from build123d import *

# Parameters (mm, degrees)
BOSS_EXTRU_1_DEPTH      = 12
ESQUISSE2_R             = 2
ENL_V_MAT_EXTRU_1_DEPTH = 28.690963204
ESQUISSE4_R             = 3.7
ENL_V_MAT_EXTRU_2_DEPTH = 17


with BuildPart() as part:
    # Esquisse1 → Boss.-Extru.1 (new, symmetric)
    with BuildSketch(Plane.XY):
        with BuildLine():
            Line((15.300968977, -0.378320662), (15.300968977, 10.466871635))
            Line((15.300968977, 10.466871635), (0, 10.466871635))
            Line((0, 10.466871635), (0, 7.5))
            ThreePointArc((0, 7.5), (5.303300859, 5.303300859), (7.5, 0))
            ThreePointArc((7.5, 0), (5.303300859, -5.303300859), (0, -7.5))
            Line((0, -7.5), (0, -9.247838393))
            Line((0, -9.247838393), (5.044275487, -9.247838393))
            Line((5.044275487, -9.247838393), (15.300968977, -0.378320662))
        make_face()
        with BuildLine():
            Line((0, 7.5), (0, 10.466871635))
            Line((0, 10.466871635), (-15.300968977, 10.466871635))
            Line((-15.300968977, 10.466871635), (-15.300968977, -0.378320662))
            Line((-15.300968977, -0.378320662), (-5.044275487, -9.247838393))
            Line((-5.044275487, -9.247838393), (0, -9.247838393))
            Line((0, -9.247838393), (0, -7.5))
            ThreePointArc((0, -7.5), (-7.5, 0), (0, 7.5))
        make_face()
    extrude(amount=BOSS_EXTRU_1_DEPTH, both=True)

    # Esquisse2 → Enlèv. mat.-Extru.1 (cut, through all)
    with BuildSketch(Plane(origin=(0, 10.466871635, 0), x_dir=(1, 0, 0), z_dir=(0, 1, 0))):
        with Locations(Location((-11.300968977, 8, 0), (0, 0, 270))):
            Circle(ESQUISSE2_R)
        with Locations(Location((-11.300968977, -8, 0), (0, 0, 270))):
            Circle(ESQUISSE2_R)
        with Locations(Location((11.300968977, -8, 0), (0, 0, 270))):
            Circle(ESQUISSE2_R)
        with Locations(Location((11.300968977, 8, 0), (0, 0, 270))):
            Circle(ESQUISSE2_R)
    extrude(amount=-ENL_V_MAT_EXTRU_1_DEPTH, mode=Mode.SUBTRACT)

    # Esquisse4 → Enlèv. mat.-Extru.2 (cut)
    with BuildSketch(Plane.XZ.offset(9.247838393)):
        with Locations(Location((-11.300968977, 8, 0), (0, 0, 270))):
            Circle(ESQUISSE4_R)
        with Locations(Location((-11.300968977, -8, 0), (0, 0, 270))):
            Circle(ESQUISSE4_R)
        with Locations(Location((11.300968977, 8, 0), (0, 0, 270))):
            Circle(ESQUISSE4_R)
        with Locations(Location((11.300968977, -8, 0), (0, 0, 270))):
            Circle(ESQUISSE4_R)
    extrude(amount=-ENL_V_MAT_EXTRU_2_DEPTH, mode=Mode.SUBTRACT)


solid = part.part
Design review of the part built by this model. Coordinates are the model's own, in mm. A direction names the side the tool comes from. Coordinates: 2 decimals unless noted, no trailing zeros. Order: outer loops, then holes, each group sorted by start corner. A loop starts at its lowest first (then second) coordinate and runs counter-clockwise, first axis right, second up. Notation, with made-up numbers: (17.5, -1) -> (27.5, -1) arc R25 cw to (27.5, 38) -> close; hole circle Ø8 at (-27.75, -23.5). An arc over 180 degrees is marked (long way). One line per item, written item: value.
1) To check wall thickness, follow probe 1 along X at (y, z) = (9.95, -8); probe 2 along Z at (x, y) = (10, 5.5); probe 3 along Z at (x, y) = (-11, 1.25). State the ranges of each line that lie inside material, in increasing order. Write a range as [from, to].
Output values:
probe 1: x = [-15.3, -13.3], [-9.3, 9.3], [13.3, 15.3]
probe 2: z = [-12, -11.46], [-4.54, 4.54], [11.46, 12]
probe 3: z = [-12, -11.69], [-4.31, 4.31], [11.69, 12]
2) We need section D-D, the plane x = -12.5. Give the boundary of the cut face in (y, z), then the cut area to 3 significant figures.
Output values:
outline: (-2.8, -12) -> (10.47, -12) -> (10.47, -9.6) -> (7.75, -9.6) -> (7.75, -11.5) -> (-2.8, -11.5) -> close; (-2.8, -4.5) -> (7.75, -4.5) -> (7.75, -6.4) -> (10.47, -6.4) -> (10.47, 6.4) -> (7.75, 6.4) -> (7.75, 4.5) -> (-2.8, 4.5) -> close; (-2.8, 11.5) -> (7.75, 11.5) -> (7.75, 9.6) -> (10.47, 9.6) -> (10.47, 12) -> (-2.8, 12) -> close
area: 153 mm2
3) We need section C-C, the plane y = -4.25. Give the boundary of the cut face in (x, z), then the cut area to 3 significant figures.
Output values:
outline: (-10.82, -12) -> (-6.18, -12) -> (-6.18, 12) -> (-10.82, 12) -> (-10.82, 11.67) arc R3.7 cw to (-10.82, 4.33) -> (-10.82, -4.33) arc R3.7 cw to (-10.82, -11.67) -> close; (6.18, -12) -> (10.82, -12) -> (10.82, -11.67) arc R3.7 cw to (10.82, -4.33) -> (10.82, 4.33) arc R3.7 cw to (10.82, 11.67) -> (10.82, 12) -> (6.18, 12) -> close
area: 151 mm2
4) Machinability: for faces 1 (the face through (0, 10.467, 0)), 2 (the face through (-7.632, 1.897, -7.518)), which of the approach directions +Z, -Z, +X, -X, +Y, -Y give a long, thin tool a straight path to every point of the face, cutting with its end or side? Answer none if there is none.
Output values:
face 1: +Z, -Z, +X, -X, +Y
face 2: -Y
5) We need section B-B, the plane z = 8. Give the boundary of the cut face in (x, y).
Output values:
outline: (-15.3, -0.38) -> (-15, -0.64) -> (-15, 7.75) -> (-13.3, 7.75) -> (-13.3, 10.47) -> (-15.3, 10.47) -> close; (-9.3, 7.75) -> (-7.6, 7.75) -> (-7.6, -7.04) -> (-5.04, -9.25) -> (5.04, -9.25) -> (7.6, -7.04) -> (7.6, 7.75) -> (9.3, 7.75) -> (9.3, 10.47) -> (-9.3, 10.47) -> close; (13.3, 7.75) -> (15, 7.75) -> (15, -0.64) -> (15.3, -0.38) -> (15.3, 10.47) -> (13.3, 10.47) -> close; hole circle Ø15 at (0, 0)
6) Clearance check with flat-ended pins moving along their axes: P1, Ø6, axis at x = -10.5, z = 9.5, coming from the -Y side; P2, Ø3.5, axis at x = -11.5, z = -8.5, coming from the -Y side; P3, Ø3.5, axis at x = 11.3, z = 8, coming from the +Y side; P4, Ø5, axis at y = -4, z = -2, coming from the +X side. State where each tip first meets the part, or that it passes through.
Output values:
P1: stops at y = -7.12
P2: stops at y = 7.75
P3: passes through
P4: stops at x = 14
7) We need section A-A, the plane z = -2.75. Give the boundary of the cut face in (x, y).
Output values:
outline: (-15.3, -0.38) -> (-5.04, -9.25) -> (5.04, -9.25) -> (15.3, -0.38) -> (15.3, 10.47) -> (-15.3, 10.47) -> close; hole circle Ø15 at (0, 0)
8) Draft analysis for pull direction X (two halves, no side actions). For faces 3 (the face through (7.69, 1.87, 8.8)), 4 (the face through (-4, 7, 12)), 5 (the face through (-9.1, -5.74, 0.17)), state which applies: +X half, -X half, draft (parallel to the pull), parting line (faces both ways), or undercut.
Output values:
face 3: undercut
face 4: draft
face 5: -X half
